Design review of the part built by this model. Coordinates are the model's own, in mm. Face numbers are marked on the shaded views. A direction names the side the tool comes from. Round coordinates to 2 decimals unless told otherwise and drop trailing zeros. Write each loop counter-clockwise with the first axis right and the second up, starting at its lowest first coordinate (ties: lowest second). Pieces come first, ordered by that corner, then holes. Notation, with made-up numbers: M 49,71.25 L 58,71.25 A3 ccw 58,75.25 Z; hole C -2,86.25 d5. An arc over 180 degrees is marked long. Use CSV: the item, a comma, the result in double quotes.
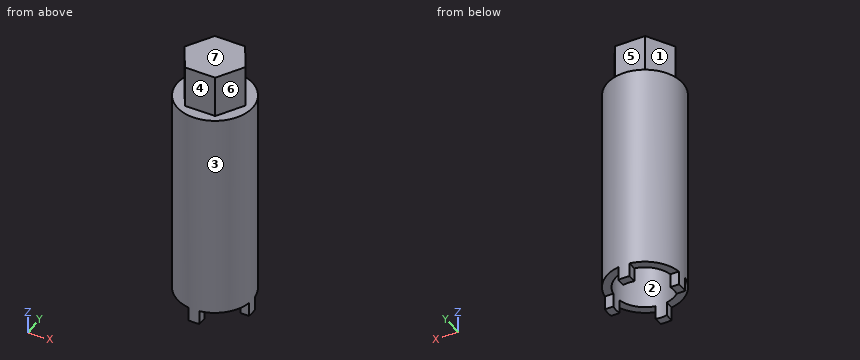
from build123d import *

# Parameters (mm, degrees)
F1_DEPTH = 15
F2_R     = 13.5
F3_DEPTH = 80
F4_R     = 10.5
F5_DEPTH = 21.6
F7_DEPTH = 5


with BuildPart() as f1:
    # F0 (on Top) → F1 (new body)
    with BuildSketch(Plane.XY):
        Polygon((-5.484828, 9.5), (-10.969655, 0), (-5.484828, -9.5), (5.484828, -9.5), (10.969655, 0), (5.484828, 9.5), align=None)
    extrude(amount=F1_DEPTH)

    # F2 (on face) → F3 (join)
    with BuildSketch(Plane(origin=(0, 0, 0), x_dir=(1, 0, 0), z_dir=(0, 0, -1))):
        Circle(F2_R)
    extrude(amount=F3_DEPTH)

    # F4 (on face) → F5 (cut)
    with BuildSketch(Plane(origin=(0, 0, -80), x_dir=(1, 0, 0), z_dir=(0, 0, -1))):
        Circle(F4_R)
    extrude(amount=-F5_DEPTH, mode=Mode.SUBTRACT)

    # F6 (on face) → F7 (cut)
    with BuildSketch(Plane(origin=(0, 0, -80), x_dir=(1, 0, 0), z_dir=(0, 0, -1))):
        with BuildLine():
            ThreePointArc((10.307764, -2), (7.424621, -7.424621), (2, -10.307764))
            Line((2, -10.307764), (2, -13.35103))
            ThreePointArc((2, -13.35103), (9.545942, -9.545942), (13.35103, -2))
            Line((13.35103, -2), (10.307764, -2))
        make_face()
        with BuildLine():
            Line((-10.307764, -2), (-13.35103, -2))
            ThreePointArc((-13.35103, -2), (-9.545942, -9.545942), (-2, -13.35103))
            Line((-2, -13.35103), (-2, -10.307764))
            ThreePointArc((-2, -10.307764), (-7.424621, -7.424621), (-10.307764, -2))
        make_face()
        with BuildLine():
            ThreePointArc((-2, 13.35103), (-9.545942, 9.545942), (-13.35103, 2))
            Line((-13.35103, 2), (-10.307764, 2))
            ThreePointArc((-10.307764, 2), (-7.424621, 7.424621), (-2, 10.307764))
            Line((-2, 10.307764), (-2, 13.35103))
        make_face()
        with BuildLine():
            ThreePointArc((13.35103, 2), (9.545942, 9.545942), (2, 13.35103))
            Line((2, 13.35103), (2, 10.307764))
            ThreePointArc((2, 10.307764), (7.424621, 7.424621), (10.307764, 2))
            Line((10.307764, 2), (13.35103, 2))
        make_face()
    extrude(amount=-F7_DEPTH, mode=Mode.SUBTRACT)


solid = f1.part
1) For pin 1 Ø1.5 at (x, z) = (-2, -54) entering from -Y; pin 2 Ø2.5 at (x, z) = (12.5, -78.5) entering from -Y; pin 3 Ø1.5 at (y, z) = (12.5, -78.5) entering from +X, all flat-tipped, find the tip position at first contact; note any pin that passes through.
Answers:
pin 1,"y = -13.44"
pin 2,"y = -2"
pin 3,"x = 2"
2) Wall thickness on line 1 along X through (y, z) = (0, -75); line 2 along Y through (x, z) = (-1.5, 10): over which ranges is each line inside the solid? List them lowest first. Write a range as [from, to].
Answers:
line 1,"[-13.5, -10.5], [10.5, 13.5]"
line 2,"[-9.5, 9.5]"
3) Add section C-C on y = -3.5. Write out the cut boundary in (x, z), then the cut area to 3 significant figures.
Answers:
outline,"M -13.04,-75 L -9.9,-75 L -9.9,-58.4 L 9.9,-58.4 L 9.9,-75 L 13.04,-75 L 13.04,0 L 8.95,0 L 8.95,15 L -8.95,15 L -8.95,0 L -13.04,0 Z"
area,"1,900 mm²"
4) The part is to be moulded in two halves that separate along Y. For the marked faces 1, 2, 3 and 4, say which applies: released by +Y, released by -Y, zero draft, split by the parting line, or undercut.
Answers:
face 1,"released by +Y"
face 2,"undercut"
face 3,"split by the parting line"
face 4,"released by -Y"
5) Machinability: for the marked faces 5, 6 and 7, which of the approach directions +Z, -Z, +X, -X, +Y, -Y give a long, thin tool a straight path to every point of the face, cutting with its end or side? Answer none if there is none.
Answers:
face 5,"+Z, +X, -X, +Y"
face 6,"+Z, +X, -Y"
face 7,"+Z, +X, -X, +Y, -Y"
6) Add section B-B on z = -60. Write out the cut boundary in (x, y).
Answers:
outline,"C 0,0 d27; hole C 0,0 d21"
7) Add section D-D on z = -16.5. Write out the cut boundary in (x, y), then the cut area to 3 significant figures.
Answers:
outline,"C 0,0 d27"
area,"573 mm²"
8) Add section A-A on x = 0. Write out the cut boundary in (y, z).
Answers:
outline,"M -13.5,-80 L -10.5,-80 L -10.5,-58.4 L 10.5,-58.4 L 10.5,-80 L 13.5,-80 L 13.5,0 L 9.5,0 L 9.5,15 L -9.5,15 L -9.5,0 L -13.5,0 Z"
